For this review, take the finished solid that the model builds, in its own axes (mm). Face numbers are marked on the shaded views. A direction names the side the tool comes from. Round coordinates to 2 decimals unless told otherwise and drop trailing zeros. Order: outer loops, then holes, each group sorted by start corner. A loop starts at its lowest first (then second) coordinate and runs counter-clockwise, first axis right, second up. Notation, with made-up numbers: M 38.5,-26 L 94.5,-26 A30 ccw 94.5,1 Z; hole C -38.75,46.25 d9. An arc over 180 degrees is marked long. Put each result on its own line as item: value.
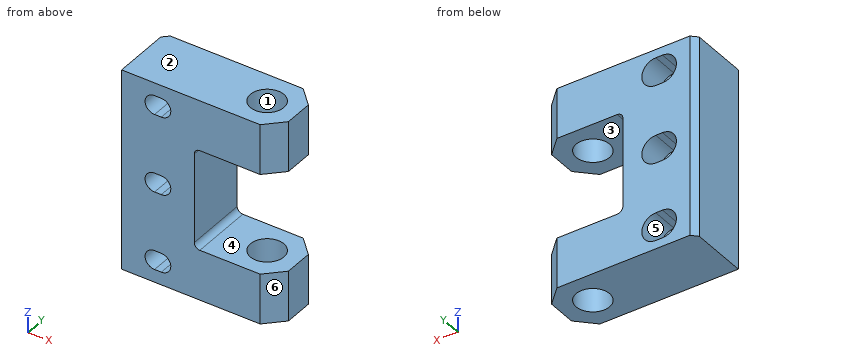
from build123d import *

# Parameters (mm, degrees)
EXTRUDE_1_DEPTH        = 56
CUT_EXTRUDE_1_REACH    = 176.806
CUT_EXTRUDE_2_DEPTH    = 24
PATTERN_LINEAR_1_COUNT = 3
PATTERN_LINEAR_1_PITCH = 70
SKETCH_4_R             = 15
CUT_EXTRUDE_3_DEPTH    = 235.215712539
CHAMFER_1_SIZE         = 5
CHAMFER_2_SIZE         = 15
FILLET_1_R             = 5


with BuildPart() as part:
    # 草图1 → 凸台-拉伸1 (new body)
    with BuildSketch(Plane(origin=(0, 0, 0), x_dir=(1, 0, 0), z_dir=(0, 1, 0))):
        Polygon((0, -90), (0, 90), (139, 90), (139, 45), (65, 45), (65, -45), (139, -45), (139, -90), align=None)
    extrude(amount=-EXTRUDE_1_DEPTH)

    # 草图2 → 切除-拉伸1 (cut, up to next)
    with BuildSketch(Plane(origin=(0, 0, 0), x_dir=(1, 0, 0), z_dir=(0, 1, 0)), mode=Mode.PRIVATE) as cut_extrude_1_sk1:
        with BuildLine():
            Line((29.5, 78.5), (35.5, 78.5))
            ThreePointArc((35.5, 78.5), (44, 70), (35.5, 61.5))
            Line((35.5, 61.5), (29.5, 61.5))
            ThreePointArc((29.5, 61.5), (21, 70), (29.5, 78.5))
        make_face()
    cut_extrude_1_tool1 = extrude(cut_extrude_1_sk1.sketch, amount=-CUT_EXTRUDE_1_REACH, mode=Mode.PRIVATE) & part.part
    cut_extrude_1 = cut_extrude_1_tool1.solids().sort_by_distance((32.5, 0, -70))[0]
    add(cut_extrude_1, mode=Mode.SUBTRACT)

    # 草图3 → 切除-拉伸2 (cut)
    with BuildSketch(Plane(origin=(0, 0, 0), x_dir=(1, 0, 0), z_dir=(0, 1, 0))):
        with BuildLine():
            Line((29.5, 57.5), (35.5, 57.5))
            ThreePointArc((35.5, 57.5), (48, 70), (35.5, 82.5))
            Line((35.5, 82.5), (29.5, 82.5))
            ThreePointArc((29.5, 82.5), (17, 70), (29.5, 57.5))
        make_face()
    cut_extrude_2 = extrude(amount=-CUT_EXTRUDE_2_DEPTH, mode=Mode.SUBTRACT)

    # 阵列(线性)1: 切除-拉伸1, 切除-拉伸2 ×3
    with Locations(*[(0, 0, i * PATTERN_LINEAR_1_PITCH) for i in range(1, PATTERN_LINEAR_1_COUNT)]):
        add(cut_extrude_1, mode=Mode.SUBTRACT)
        add(cut_extrude_2, mode=Mode.SUBTRACT)

    # 草图4 → 切除-拉伸3 (cut, through all)
    with BuildSketch(Plane.XY.offset(90)):
        with Locations((111, -28)):
            Circle(SKETCH_4_R)
    extrude(amount=-CUT_EXTRUDE_3_DEPTH, mode=Mode.SUBTRACT)

    # 倒角1
    chamfer_1_edges = [part.edges().sort_by_distance(p)[0] for p in [
        (0, 0, 0),
    ]]
    chamfer(chamfer_1_edges, length=CHAMFER_1_SIZE)

    # 倒角2
    chamfer_2_edges = [part.edges().sort_by_distance(p)[0] for p in [
        (139, -56, 67.5),
        (139, -56, -67.5),
        (139, 0, -67.5),
        (139, 0, 67.5),
    ]]
    chamfer(chamfer_2_edges, length=CHAMFER_2_SIZE)

    # 圆角1
    fillet_1_edges = [part.edges().sort_by_distance(p)[0] for p in [
        (65, -28, -45),
        (65, -28, 45),
    ]]
    fillet(fillet_1_edges, radius=FILLET_1_R)


solid = part.part
(1) For the marked faces 4, 5 and 6, list the 3-axis set-ups (+Z, -Z, +X, -X, +Y, -Y) from which the entire face can be reached by the end or side of a thin tool; tool diameter is ignored.
A:
face 4: +X, +Y, -Y
face 5: +Y
face 6: +Z, -Z, +X, -Y
(2) Draft analysis for pull direction Z (two halves, no side actions). For the marked faces 1, 2 and 3, state which applies: released by +Z, released by -Z, zero draft, split by the parting line, or undercut.
A:
face 1: zero draft
face 2: released by +Z
face 3: undercut
(3) Add section C-C on z = -70. Give the boundary of the cut face in (x, y).
A:
outline: M 0,-56 L 21,-56 L 21,-24 L 17,-24 L 17,0 L 5,0 L 0,-5 Z; M 44,-56 L 124,-56 L 139,-41 L 139,-15 L 124,0 L 48,0 L 48,-24 L 44,-24 Z; hole C 111,-28 d30
(4) Add section D-D on x = 111. Give the boundary of the cut face in (y, z).
A:
outline: M -56,-90 L -43,-90 L -43,-45 L -56,-45 Z; M -56,45 L -43,45 L -43,90 L -56,90 Z; M -13,-90 L 0,-90 L 0,-45 L -13,-45 Z; M -13,45 L 0,45 L 0,90 L -13,90 Z
(5) To check wall thickness, follow L1, parallel to Y at x = 111, z = -56; L2, parallel to Z at x = 77, y = -13.5; L3, parallel to X at y = -53, z = 11.5. State the ranges of each line that lie inside material, in increasing order.
A:
L1: y = -56 to -43, -13 to 0
L2: z = -90 to -45, 45 to 90
L3: x = 0 to 65
(6) Add section B-B on x = 130.5. Give the boundary of the cut face in (y, z).
A:
outline: M -49.5,-90 L -6.5,-90 L -6.5,-45 L -49.5,-45 Z; M -49.5,45 L -6.5,45 L -6.5,90 L -49.5,90 Z
(7) Insertion check: pin 1 Ø8 at (x, z) = (113, -42) entering from -Y; pin 2 Ø4 at (y, z) = (-7.5, -48) entering from +X; pin 3 Ø8 at (y, z) = (-45.5, 12.5) entering from +X; pin 4 Ø7.5 at (x, z) = (39, -6) entering from +Y. Each pin has a flat end and moves straight along its axis. Give the tip position at first contact, or say it passes through.
A:
pin 1: stops at y = -56
pin 2: stops at x = 133.5
pin 3: stops at x = 65
pin 4: stops at y = -24
(8) Add section A-A on y = -28. State how many separate pieces and enclosed holes the cut face has, then the cut area to 3 significant figures.
A:
separate pieces: 3
enclosed holes: 3
area: 14,700 mm2
